Could you check a few things on this model? Use its own coordinates, in mm. A direction names the side the tool comes from. Coordinates: 2 decimals unless noted, no trailing zeros. Write each loop counter-clockwise with the first axis right and the second up, starting at its lowest first coordinate (ties: lowest second). Pieces come first, ordered by that corner, then holes.
Item 1: If I drill on probe 1 along Z at (x, y) = (-11, 14); probe 2 along X at (y, z) = (66.5, -14.5); probe 3 along Y at (x, z) = (46, 0), over which ranges is the centre line in solid material (lowest first)?
Item 2: Thinking about a two-plate mould opening in X: for faces 1 (the flat face through (-100, 57, 1)), 2 (the flat face through (-1, 59, -82)), 3 (the flat face through (-102, 59, 1)), 4 (the flat face through (102, 59, 1)), which applies, +X half, -X half, draft (parallel to the pull), parting line (faces both ways), or undercut?
Item 3: I want a section at B-B on z = -54. Please give me the cut outline in (x, y).
Item 4: I want a section at A-A on y = 73. Please give me the cut outline in (x, z).
Item 5: For P1, Ø3, axis at x = -16, z = 52, coming from the -Y side, with a flat end and sliding along its axis, tell me the tip position at first contact or that it passes through.
Item 6: I want a section at C-C on x = -19.5. Please give me the cut outline in (y, z).
Item 7: Which directions (+Z, -Z, +X, -X, +Y, -Y) give clear straight access to the entire face, cutting with the end or side of a thin tool? Please do faces 5 (the flat face through (-1, 57, 80)), 6 (the flat face through (-1, 120, -1)).
from build123d import *

# Parameters (mm, degrees)
SKETCH4_W           = 204
SKETCH4_H           = 164
BOSS_EXTRUDE3_DEPTH = 120
SKETCH5_W           = 200
SKETCH5_H           = 160
CUT_EXTRUDE2_DEPTH  = 116


with BuildPart() as part:
    # Sketch4 → Boss-Extrude3 (new body)
    with BuildSketch(Plane(origin=(0, 0, 0), x_dir=(1, 0, 0), z_dir=(0, 1, 0))):
        Rectangle(SKETCH4_W, SKETCH4_H)
    extrude(amount=BOSS_EXTRUDE3_DEPTH)

    # Sketch5 → Cut-Extrude2 (cut)
    with BuildSketch(Plane(origin=(0, 0, 0), x_dir=(1, 0, 0), z_dir=(0, 1, 0))):
        Rectangle(SKETCH5_W, SKETCH5_H)
    extrude(amount=CUT_EXTRUDE2_DEPTH, mode=Mode.SUBTRACT)


solid = part.part
Response values:
1. probe 1: z = -82 to -80, 80 to 82
1. probe 2: x = -102 to -100, 100 to 102
1. probe 3: y = 116 to 120
2. face 1: undercut
2. face 2: draft
2. face 3: -X half
2. face 4: +X half
3. outline: (-102, 0) - (-100, 0) - (-100, 116) - (100, 116) - (100, 0) - (102, 0) - (102, 120) - (-102, 120) - close
4. outline: (-102, -82) - (102, -82) - (102, 82) - (-102, 82) - close; hole (-100, -80) - (100, -80) - (100, 80) - (-100, 80) - close
5. P1: stops at y = 116
6. outline: (0, -82) - (120, -82) - (120, 82) - (0, 82) - (0, 80) - (116, 80) - (116, -80) - (0, -80) - close
7. face 5: -Y
7. face 6: +Z, -Z, +X, -X, +Y
